from build123d import *

# Parameters (mm, degrees)
F1_DEPTH = 6
F3_DEPTH = 2
F4_R     = 2.25
F5_DEPTH = 8.001
F6_R     = 3.75
F7_DEPTH = 2
F8_SIZE  = 3


with BuildPart() as f1:
    # F0 (on Top) → F1 (new body)
    with BuildSketch(Plane.XY):
        Polygon((0, 40), (0, 0), (40, 0), (40, 20), (20, 20), (20, 40), align=None)
    extrude(amount=F1_DEPTH)

    # F2 (on face) → F3 (join)
    with BuildSketch(Plane.XY.offset(6)):
        Polygon((12.71, 40), (7.29, 40), (7.29, 20), (10, 20), (12.71, 20), align=None)
        Polygon((40, 7.29), (40, 12.71), (20, 12.71), (20, 10), (20, 7.29), align=None)
    extrude(amount=F3_DEPTH)

    # F4 (on face) → F5 (cut, through all)
    with BuildSketch(Plane(origin=(0, 0, 0), x_dir=(1, 0, 0), z_dir=(0, 0, -1))):
        with Locations((10, -30)):
            Circle(F4_R)
        with Locations((10, -10)):
            Circle(F4_R)
        with Locations((30, -10)):
            Circle(F4_R)
    extrude(amount=-F5_DEPTH, mode=Mode.SUBTRACT)

    # F6 (on face) → F7 (cut)
    with BuildSketch(Plane(origin=(0, 0, 0), x_dir=(1, 0, 0), z_dir=(0, 0, -1))):
        with Locations((10, -10)):
            Circle(F6_R)
        with Locations((30, -10)):
            Circle(F6_R)
        with Locations((10, -30)):
            Circle(F6_R)
    extrude(amount=-F7_DEPTH, mode=Mode.SUBTRACT)

    # F8
    f8_edges = [f1.edges().sort_by_distance(p)[0] for p in [
        (20, 0, 0),
        (0, 20, 0),
        (20, 30, 0),
        (30, 20, 0),
        (40, 10, 0),
        (10, 40, 0),
    ]]
    chamfer(f8_edges, length=F8_SIZE)


solid = f1.part
Source: CAD feature listing. Evaluate the final solid. Frame: model axes, mm. A direction names the side the tool comes from. Give positions to 0.01 mm unless a question says otherwise; leave off trailing zeros. Write each loop counter-clockwise with the first axis right and the second up, starting at its lowest first coordinate (ties: lowest second). Pieces come first, ordered by that corner, then holes. Notation, with made-up numbers: M -2,2 L 42,2 A24 cw 42,31 Z; hole C 38,64 d5. An arc over 180 degrees is marked long. Return JSON: item names as keys, results as strings. Group by question number.
1) Draft query along X for faces 1 (the face through (31.21, 8.103, 4.958)), 2 (the face through (7.29, 30, 7)), 3 (the face through (10, 38, 1)). Return one class per face: released by +X, released by -X, zero draft, split by the parting line, or undercut.
2) Cut plane C-C, the plane x = 10. Output: boundary loops of the cut face in (y, z).
3) Set-up query: faces 4 (the face through (19, 28, 2)), 5 (the face through (7.236, 27.466, 0.986)), 6 (the face through (30, 7.29, 7)). Return all of +Z, -Z, +X, -X, +Y, -Y with unobstructed straight access to the full face (end or side cutting, diameter ignored); none if empty.
4) Ray query, L1, parallel to Y at x = 10, z = 4.05; L2, parallel to X at y = 10, z = 1. Return the intervals inside material, ascending.
5) Cut plane D-D, the plane z = 5. Output: boundary loops of the cut face in (x, y), then the cut area to 3 significant figures.
6) Cut plane A-A, the plane x = 30. Output: boundary loops of the cut face in (y, z), then the cut area to 3 significant figures.
7) First-contact query: pin 1 Ø2 at (y, z) = (33.5, 6.5) entering from -X; pin 2 Ø5 at (x, y) = (10, 30) entering from -Z; pin 3 Ø0.6 at (x, z) = (35, 7) entering from -Y; pin 4 Ø1 at (y, z) = (26.5, 7) entering from +X. Flat tips, straight axial feed; report the tip coordinate or a pass-through.
Data:
{
 "1": {"face 1": "undercut", "face 2": "released by -X", "face 3": "zero draft"},
 "2": {"outline": "M 0,3 L 3,0 L 6.25,0 L 6.25,2 L 7.75,2 L 7.75,6 L 0,6 Z; M 12.25,2 L 13.75,2 L 13.75,0 L 26.25,0 L 26.25,2 L 27.75,2 L 27.75,8 L 20,8 L 20,6 L 12.25,6 Z; M 32.25,2 L 33.75,2 L 33.75,0 L 37,0 L 40,3 L 40,8 L 32.25,8 Z"},
 "3": {"face 4": "-Z, +X, +Y", "face 5": "-Z", "face 6": "+Z, +X, -X, -Y"},
 "4": {"L1": "y = 0 to 7.75, 12.25 to 27.75, 32.25 to 40", "L2": "x = 2 to 6.25, 13.75 to 26.25, 33.75 to 38"},
 "5": {"outline": "M 0,0 L 40,0 L 40,20 L 20,20 L 20,40 L 0,40 Z; hole C 10,10 d4.5; hole C 10,30 d4.5; hole C 30,10 d4.5", "area": "1,150 mm²"},
 "6": {"outline": "M 0,3 L 3,0 L 6.25,0 L 6.25,2 L 7.75,2 L 7.75,8 L 7.29,8 L 7.29,6 L 0,6 Z; M 12.25,2 L 13.75,2 L 13.75,0 L 17,0 L 20,3 L 20,6 L 12.71,6 L 12.71,8 L 12.25,8 Z", "area": "79.8 mm²"},
 "7": {"pin 1": "stops at x = 0", "pin 2": "stops at z = 2", "pin 3": "stops at y = 7.29", "pin 4": "stops at x = 12.71"}
}
